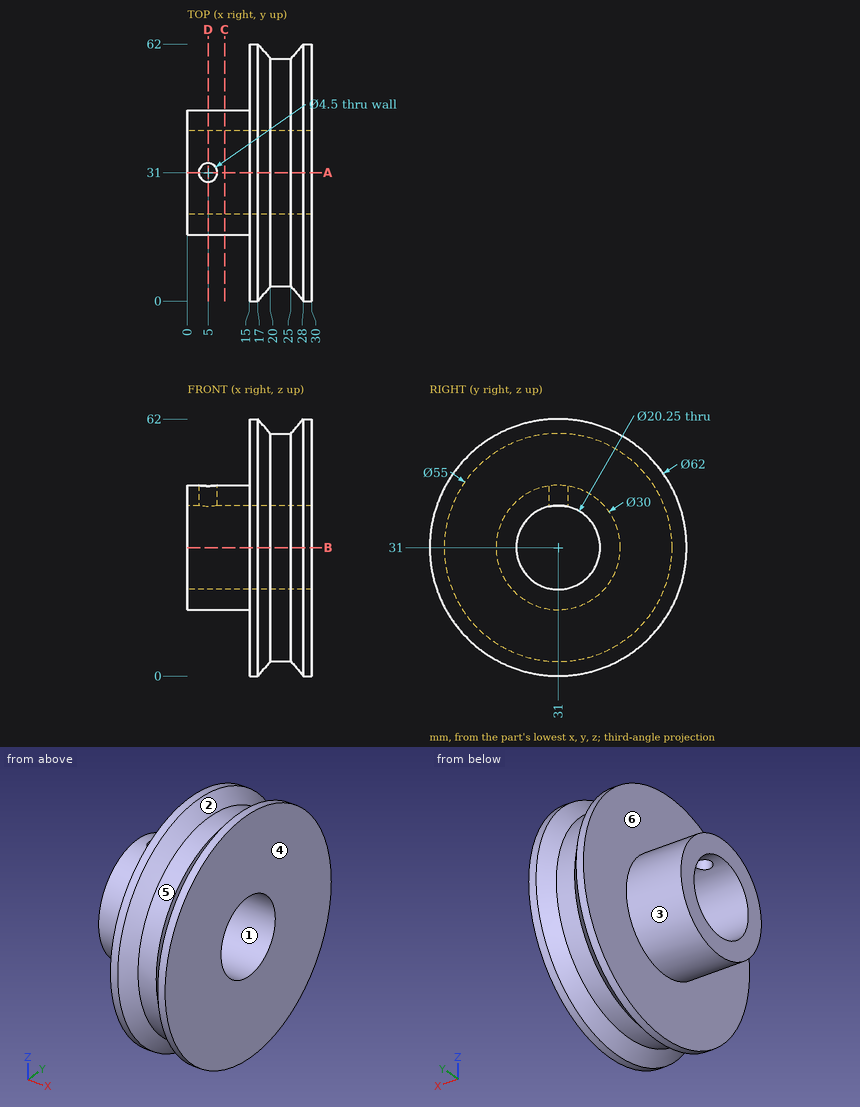
Input: dimensioned drawing with shaded views. Units: mm. Origin: part minimum x, y, z. A direction names the side the tool comes from. Give positions to 0.01 mm unless a question says otherwise; leave off trailing zeros. Write each loop counter-clockwise with the first axis right and the second up, starting at its lowest first coordinate (ties: lowest second). Pieces come first, ordered by that corner, then holes.
1. First-contact query: pin 1 (5 mm diameter, centred on x = 17.5, z = 44, fed in from +Y); pin 2 (1.5 mm diameter, centred on x = 16, y = 51, fed in from -Z); pin 3 (1 mm diameter, centred on x = 20, z = 23.5, fed in from +Y). Flat tips, straight axial feed; report the tip coordinate or a pass-through.
2. Access query for the marked faces 1, 2 and 3. Directions: +Z, -Z, +X, -X, +Y, -Y. A direction counts if a zero-diameter tool reaches every point of the face in a straight line with its end or side. Return the directions, or none.
3. Pull-direction query (X, two-part tool) for the marked faces 4, 5 and 6; classes: +X half, -X half, draft (parallel to the pull), parting line (faces both ways), or undercut.
4. Material intervals for line 1 along Y through (x, z) = (14, 30.5); line 2 along X through (y, z) = (31, 44.15); line 3 along Z through (x, y) = (14, 31) (3 decimals), sorted ascending.
5. Section query B-B (z = 31). Return the cut outline in (x, y) (3 decimals).
6. Section query D-D (x = 5). Return the cut outline in (y, z) (3 decimals), then the cut area to 3 significant figures.
7. Section query A-A (y = 31). Return the cut outline in (x, z) (3 decimals).
8. Section query C-C (x = 9). Return the cut outline in (y, z) (3 decimals), then the cut area to 3 significant figures.
Output values:
1. pin 1: stops at y = 60.15
1. pin 2: stops at z = 6.7
1. pin 3: stops at y = 58.08
2. face 1: +X, -X
2. face 2: none
2. face 3: -X
3. face 4: +X half
3. face 5: undercut
3. face 6: -X half
4. line 1: y = 16.01 to 20.89, 41.11 to 45.99
4. line 2: x = 0 to 2.75, 7.25 to 30
4. line 3: z = 16 to 20.875, 41.125 to 46
5. outline: (0, 16) - (15, 16) - (15, 0) - (17, 0) - (20, 3.5) - (25, 3.5) - (28, 0) - (30, 0) - (30, 20.875) - (0, 20.875) - close; (0, 41.125) - (30, 41.125) - (30, 62) - (28, 62) - (25, 58.5) - (20, 58.5) - (17, 62) - (15, 62) - (15, 46) - (0, 46) - close
6. outline: (28.75, 40.872) - (28.75, 45.83) arc R15 ccw (long way) to (33.25, 45.83) - (33.25, 40.872) arc R10.125 cw (long way) to start
6. area: 363 mm2
7. outline: (0, 16) - (15, 16) - (15, 0) - (17, 0) - (20, 3.5) - (25, 3.5) - (28, 0) - (30, 0) - (30, 20.875) - (0, 20.875) - close; (0, 41.125) - (2.75, 41.125) - (2.75, 46) - (0, 46) - close; (7.25, 41.125) - (30, 41.125) - (30, 62) - (28, 62) - (25, 58.5) - (20, 58.5) - (17, 62) - (15, 62) - (15, 46) - (7.25, 46) - close
8. outline: circle Ø30 at (31, 31); hole circle Ø20.25 at (31, 31)
8. area: 385 mm2
